Model file for the job. Use its own axes, mm. Face numbers are marked on the shaded views. A direction names the side the tool comes from. Give positions to 0.01 mm unless a question says otherwise; leave off trailing zeros. Loops run counter-clockwise (first coordinate to the right, second up) from the corner with the lowest first, then second, coordinate; pieces in that order, holes last. Notation, with made-up numbers: (-25.75, 10.5) -> (-4.75, 10.5) arc R23 ccw to (-4.75, 25.5) -> close; hole circle Ø3 at (77.25, 58). An arc over 180 degrees is marked (long way). Use CSV: the item, a comma, the result in double quotes. Start each with the question number.
(1) 3-axis set-ups, long thin cutter, end or side, ignore diameter. For the marked faces 4, 5, 6 and 7: which of +Z, -Z, +X, -X, +Y, -Y reach the whole face in a straight line?
(2) Drill centre lines: probe 1 along Y at (x, z) = (6.5, -4.5); probe 2 along X at (y, z) = (2, -5.25); probe 3 along X at (y, z) = (20.25, -5.5). Where is each one in solid material? Low to high.
(3) Cut at D-D on z = -1. Write the cut outline in (x, y) (3 decimals), then the cut area to 3 significant figures.
(4) Pull direction X, two halves, no side cores. Call the marked faces 1, 2 and 3: pulls with the +X half, pulls with the -X half, needs draft (parallel to the pull), parting line crosses it, or undercut.
(5) Cut at C-C on x = -13.75. Write the cut outline in (y, z), then the cut area to 3 significant figures.
(6) Flat gauge pins, fed straight in: pin 1 (2 mm diameter, centred on x = 0, y = 7, fed in from -Z) (3 decimals); pin 2 (2 mm diameter, centred on x = -14.5, z = -1, fed in from +Y); pin 3 (2 mm diameter, centred on y = 19, z = -0.5, fed in from +X). Where does each tip first touch, or does it go through?
(7) Cut at B-B on z = 5. Write the cut outline in (x, y).
(8) Cut at A-A on y = 9.5. Write the cut outline in (x, z) (3 decimals).
from build123d import *

# Parameters (mm, degrees)
SKETCH1_W                 = 35
SKETCH1_H                 = 12
BOSS_EXTRUDE1_DEPTH       = 10
SKETCH2_W                 = 20
SKETCH2_H                 = 12
BOSS_EXTRUDE2_DEPTH       = 25
CUT_EXTRUDE1_DEPTH        = 21.65
SKETCH6_W                 = 10.63
SKETCH6_H                 = 8.25
CUT_EXTRUDE2_DEPTH        = 3.35
SKETCH8_R                 = 1
BOSS_EXTRUDE3_DEPTH       = 21.65
CUT_EXTRUDE3_DEPTH        = 0.5
CUT_EXTRUDE3_DEPTH_BACK   = 1.5
SKETCH9_W                 = 13.86
SKETCH9_H                 = 10.85
TAP_DRILL_FOR_8_32_TAP1_D = 3.4544


with BuildPart() as part:
    # Sketch1 → Boss-Extrude1 (new body)
    with BuildSketch(Plane(origin=(0, 0, 0), x_dir=(1, 0, 0), z_dir=(0, 1, 0))):
        Rectangle(SKETCH1_W, SKETCH1_H)
    extrude(amount=BOSS_EXTRUDE1_DEPTH)

    # Sketch2 → Boss-Extrude2 (add)
    with BuildSketch(Plane(origin=(0, 0, 0), x_dir=(1, 0, 0), z_dir=(0, 1, 0))):
        Rectangle(SKETCH2_W, SKETCH2_H)
    extrude(amount=BOSS_EXTRUDE2_DEPTH)

    # Sketch5 → Cut-Extrude1 (cut)
    with BuildSketch(Plane(origin=(0, 0, 0), x_dir=(1, 0, 0), z_dir=(0, 1, 0))):
        with BuildLine():
            Line((6.93, 6), (6.93, -2.365))
            ThreePointArc((6.93, -2.365), (6.563883476, -3.248883476), (5.68, -3.615))
            Line((5.68, -3.615), (-5.68, -3.615))
            ThreePointArc((-5.68, -3.615), (-6.563883476, -3.248883476), (-6.93, -2.365))
            Line((-6.93, -2.365), (-6.93, 6))
            Line((-6.93, 6), (6.93, 6))
        make_face()
    extrude(amount=CUT_EXTRUDE1_DEPTH, mode=Mode.SUBTRACT)

    # Sketch6 → Cut-Extrude2 (cut)
    with BuildSketch(Plane(origin=(0, 25, 0), x_dir=(1, 0, 0), z_dir=(0, 1, 0))):
        with Locations((0, 1.875)):
            Rectangle(SKETCH6_W, SKETCH6_H)
    extrude(amount=-CUT_EXTRUDE2_DEPTH, mode=Mode.SUBTRACT)

    # Sketch8 → Boss-Extrude3 (add)
    with BuildSketch(Plane.XZ):
        with Locations((-6.93, -4.1762495)):
            Circle(SKETCH8_R)
        with Locations((6.93, -4.1762495)):
            Circle(SKETCH8_R)
    extrude(amount=-BOSS_EXTRUDE3_DEPTH)

    # Sketch9 → Cut-Extrude3 (cut, two sides: drawn at the far end of the back side and taken through both)
    with BuildSketch(Plane.XZ.offset(-7.21).offset(-CUT_EXTRUDE3_DEPTH_BACK)):
        Rectangle(SKETCH9_W, SKETCH9_H)
    extrude(amount=CUT_EXTRUDE3_DEPTH + CUT_EXTRUDE3_DEPTH_BACK, mode=Mode.SUBTRACT)

    # Tap Drill for #8-32 Tap1 (through all)
    with Locations(Plane(origin=(0, 10, 0), x_dir=(1, 0, 0), z_dir=(0, 1, 0))):
        with Locations((-13.75, 0), (13.75, 0)):
            Hole(TAP_DRILL_FOR_8_32_TAP1_D / 2)


solid = part.part
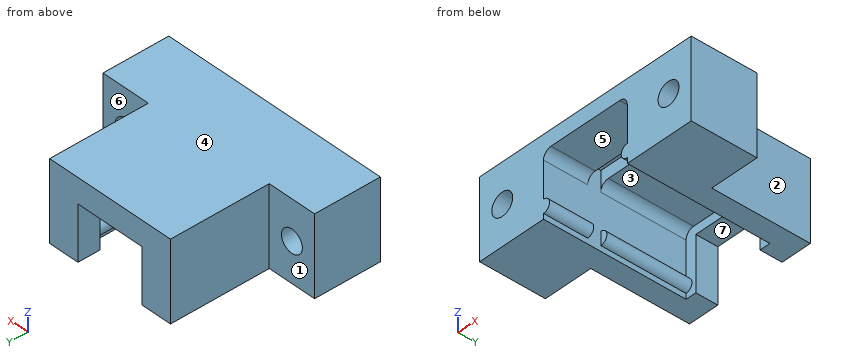
Check result:
1,face 4,"+Z, +X, -X, +Y, -Y"
1,face 5,"-Z, -Y"
1,face 6,"+Z, -Z, +X, +Y"
1,face 7,"-Z, +Y, -Y"
2,probe 1,"0 to 6.71, 8.71 to 25"
2,probe 2,"-17.5 to -6.93, 6.93 to 17.5"
2,probe 3,"-10 to -6.93, 6.93 to 10"
3,outline,"(-17.5, 0) -> (-15.158, 0) -> (-15.158, 10) -> (-17.5, 10) -> close; (-12.342, 0) -> (-6.93, 0) -> (-6.93, 21.65) -> (-5.315, 21.65) -> (-5.315, 25) -> (-10, 25) -> (-10, 10) -> (-12.342, 10) -> close; (5.315, 21.65) -> (6.93, 21.65) -> (6.93, 0) -> (12.342, 0) -> (12.342, 10) -> (10, 10) -> (10, 25) -> (5.315, 25) -> close; (15.158, 0) -> (17.5, 0) -> (17.5, 10) -> (15.158, 10) -> close"
3,area,"258 mm²"
4,face 1,"needs draft"
4,face 2,"pulls with the +X half"
4,face 3,"undercut"
5,outline,"(0, -6) -> (10, -6) -> (10, -1.73) -> (0, -1.73) -> close; (0, 1.73) -> (10, 1.73) -> (10, 6) -> (0, 6) -> close"
5,area,"85.5 mm²"
6,pin 1,"z = 3.615"
6,pin 2,"y = 10"
6,pin 3,"x = 10"
7,outline,"(-17.5, 0) -> (17.5, 0) -> (17.5, 10) -> (10, 10) -> (10, 25) -> (-10, 25) -> (-10, 10) -> (-17.5, 10) -> close; hole (-6.93, 6.71) -> (6.93, 6.71) -> (6.93, 8.71) -> (-6.93, 8.71) -> close"
8,outline,"(-17.5, -6) -> (-6.93, -6) -> (-6.93, -5.176) arc R1 ccw to (-6.93, -3.176) -> (-6.93, 2.365) arc R1.25 cw to (-5.68, 3.615) -> (5.68, 3.615) arc R1.25 cw to (6.93, 2.365) -> (6.93, -3.176) arc R1 ccw to (6.93, -5.176) -> (6.93, -6) -> (17.5, -6) -> (17.5, 6) -> (-17.5, 6) -> close; hole circle Ø3.454 at (-13.75, 0); hole circle Ø3.454 at (13.75, 0)"
